Geometry check sheet. Reference: the model listing, model coordinates, mm. A direction names the side the tool comes from. Coordinates: 2 decimals unless noted, no trailing zeros. Write each loop counter-clockwise with the first axis right and the second up, starting at its lowest first coordinate (ties: lowest second). Pieces come first, ordered by that corner, then holes.
from build123d import *

# Parameters (mm, degrees)
SKETCH1_W               = 27.191844216
SKETCH1_H               = 9.407407408
BOSS_EXTRUDE1_DEPTH     = 16.51
SKETCH1_3_W             = 12.7
SKETCH1_3_H             = 9.407407408
BOSS_EXTRUDE2_DEPTH     = 5.08
CUT_EXTRUDE1_DEPTH      = 20.828
CUT_EXTRUDE1_DEPTH_BACK = 20.828
SKETCH2_W               = 5.594013652
SKETCH2_H               = 17.651209439


with BuildPart() as part:
    # Sketch1 → Boss-Extrude1 (new body)
    with BuildSketch(Plane(origin=(0, 0, 0), x_dir=(0, 0, -1), z_dir=(1, 0, 0))):
        with Locations((-11.239440409, 3.175)):
            Rectangle(SKETCH1_W, SKETCH1_H)
    extrude(amount=BOSS_EXTRUDE1_DEPTH)

    # Sketch1<3> → Boss-Extrude2 (add)
    with BuildSketch(Plane(origin=(0, 0, 0), x_dir=(0, 0, -1), z_dir=(1, 0, 0))):
        with Locations((-31.185362517, 3.175)):
            Rectangle(SKETCH1_3_W, SKETCH1_3_H)
        with Locations((8.706481699, 3.175)):
            Rectangle(SKETCH1_3_W, SKETCH1_3_H)
    extrude(amount=BOSS_EXTRUDE2_DEPTH)

    # Sketch2 → Cut-Extrude1 (cut, two sides: drawn at the far end of the back side and taken through both)
    with BuildSketch(Plane(origin=(0, 0, 0), x_dir=(1, 0, 0), z_dir=(0, 1, 0)).offset(-CUT_EXTRUDE1_DEPTH_BACK)):
        with Locations((2.797006826, -11.06204132)):
            Rectangle(SKETCH2_W, SKETCH2_H)
    extrude(amount=CUT_EXTRUDE1_DEPTH + CUT_EXTRUDE1_DEPTH_BACK, mode=Mode.SUBTRACT)


solid = part.part
1. Sectioned sample at B-B, the plane y = 1.5. Record the boundary of the cut face in (x, z).
Computed values:
outline: (0, -15.06) - (5.08, -15.06) - (5.08, -2.36) - (16.51, -2.36) - (16.51, 24.84) - (5.08, 24.84) - (5.08, 37.54) - (0, 37.54) - (0, 19.89) - (5.59, 19.89) - (5.59, 2.24) - (0, 2.24) - close
2. Draft check along Z on faces 1 (the flat face through (5.594, 3, 11)), 2 (the flat face through (3, 3, 2.236)), 3 (the flat face through (3, 3, 37.535)), 4 (the flat face through (11, 3, -2.356)). Enter one of: released by +Z, released by -Z, zero draft, split by the parting line, or undercut.
Computed values:
face 1: undercut
face 2: undercut
face 3: released by +Z
face 4: released by -Z
3. Gauge pin test, flat ends, axial feed: pin 1 Ø1.5 at (x, y) = (14, 6.5) entering from +Z; pin 2 Ø4.5 at (y, z) = (2.5, -5.5) entering from +X; pin 3 Ø4.5 at (y, z) = (4, 9.5) entering from -X. Record the tip position at first contact, or that the pin passes through.
Computed values:
pin 1: stops at z = 24.84
pin 2: stops at x = 5.08
pin 3: stops at x = 5.59
4. Access from +Z, -Z, +X, -X, +Y, -Y to the whole of each face (thin tool, end or side, straight path). Record for faces 5 (the flat face through (3, 3, 19.888)), 6 (the flat face through (5.08, 3, 31)), 7 (the flat face through (5.08, 3, -9)).
Computed values:
face 5: -X, +Y, -Y
face 6: +Z, +X, +Y, -Y
face 7: -Z, +X, +Y, -Y
5. Sectioned sample at C-C, the plane z = 4.5. Record the boundary of the cut face in (x, y).
Computed values:
outline: (5.59, -1.53) - (16.51, -1.53) - (16.51, 7.88) - (5.59, 7.88) - close
6. Sectioned sample at D-D, the plane x = 14. Record the boundary of the cut face in (y, z), and give its area (3 significant figures).
Computed values:
outline: (-1.53, -2.36) - (7.88, -2.36) - (7.88, 24.84) - (-1.53, 24.84) - close
area: 256 mm2
7. Thickness scan on line 1 along Z through (x, y) = (4.25, 7.75); line 2 along Z through (x, y) = (14.75, 5); line 3 along X through (y, z) = (4.75, 29). Record the ranges inside material, lowest first.
Computed values:
line 1: z = -15.06 to 2.24, 19.89 to 37.54
line 2: z = -2.36 to 24.84
line 3: x = 0 to 5.08
8. Sectioned sample at A-A, the plane x = 1.5. Record the boundary of the cut face in (y, z), and give its area (3 significant figures).
Computed values:
outline: (-1.53, -15.06) - (7.88, -15.06) - (7.88, 2.24) - (-1.53, 2.24) - close; (-1.53, 19.89) - (7.88, 19.89) - (7.88, 37.54) - (-1.53, 37.54) - close
area: 329 mm2
